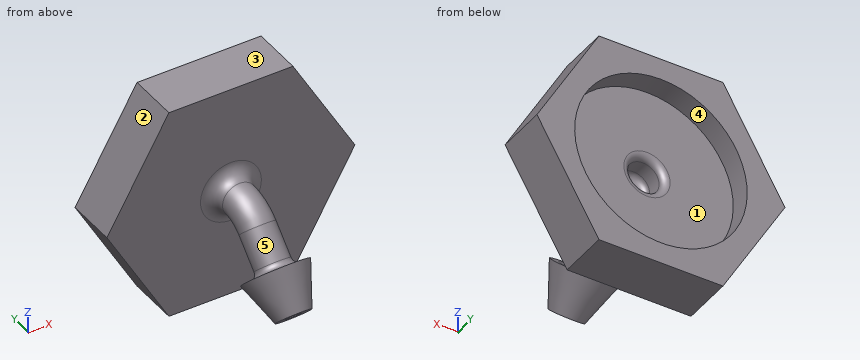
```python
from build123d import *

# Parameters (mm, degrees)
MAINHOLDER_DEPTH   = 7.5
SKETCH12_R         = 12.75
MAGNETCUTOUT_DEPTH = 3.28
MAGNETHOLE_REACH   = 26.614
SKETCH13_R         = 2.415
DRAINOPENING_R     = 2.5
DRAINOPENING_R_2   = 1.125
DRAINBASEFILLET_R  = 2
BARBBASEFILLET_R   = 1
DRAINOPENFILLET_R  = 1
MAGNETFILLET_R     = 1


with BuildPart() as part:
    # Sketch11 → MainHolder (new body)
    with BuildSketch(Plane(origin=(0, 0, 0), x_dir=(1, 0, 0), z_dir=(0, 1, 0))):
        Polygon((18.330871047, 0), (9.165435523, 15.875), (-9.165435523, 15.875), (-18.330871047, 0), (-9.165435523, -15.875), (9.165435523, -15.875), align=None)
    extrude(amount=MAINHOLDER_DEPTH)

    # Sketch12 → MagnetCutout (cut)
    with BuildSketch(Plane(origin=(0, 7.5, 0), x_dir=(1, 0, 0), z_dir=(0, 1, 0))):
        with Locations(Location((0, 0, 0), (0, 0, 270))):
            Circle(SKETCH12_R)
    extrude(amount=-MAGNETCUTOUT_DEPTH, mode=Mode.SUBTRACT)

    # Sketch13 → MagnetHole (cut, up to next)
    with BuildSketch(Plane(origin=(0, 4.22, 0), x_dir=(1, 0, 0), z_dir=(0, 1, 0)), mode=Mode.PRIVATE) as magnethole_sk1:
        with Locations(Location((0, 0, 0), (0, 0, 270))):
            Circle(SKETCH13_R)
    magnethole_tool1 = extrude(magnethole_sk1.sketch, amount=-MAGNETHOLE_REACH, mode=Mode.PRIVATE) & part.part
    add(magnethole_tool1.solids().sort_by_distance((0, 4.22, 0))[0], mode=Mode.SUBTRACT)

    # Drain: sweep along a path in DrainPath
    with BuildLine(Plane(origin=(0, 0, 0), x_dir=(0, 0, -1), z_dir=(1, 0, 0))) as drain_path:
        Line((0, 0), (0, -2))
        ThreePointArc((0, -2), (0.456722805, -4.296100594), (1.757359313, -6.242640687))
        Line((1.757359313, -6.242640687), (10.242640687, -14.727922061))
    # DrainOpening → Drain (sweep)
    with BuildSketch(Plane.XZ):
        Circle(DRAINOPENING_R)
        Circle(DRAINOPENING_R_2, mode=Mode.SUBTRACT)
    sweep(path=drain_path.line)

    # BarbOutline → Barb (revolve)
    with BuildSketch(Plane(origin=(0, 0, 0), x_dir=(0, -0.7071067811865461, -0.7071067811865489), z_dir=(-1, 0, 0)), mode=Mode.PRIVATE) as barb_sk:
        Polygon((17.656854249, 0.671572875), (11.656854249, 0.671572875), (11.656854249, -1.578427125), align=None)
    revolve(barb_sk.sketch.rotate(Axis((0, -5.447145558, -0.961864184), (0, -0.7071067811865461, -0.707106781186549)), 180), axis=Axis((0, -5.447145558, -0.961864184), (0, -0.7071067811865461, -0.707106781186549)))

    # DrainBaseFillet
    drainbasefillet_edges = [part.edges().sort_by_distance(p)[0] for p in [
        (-2.5, 0, 0),
    ]]
    fillet(drainbasefillet_edges, radius=DRAINBASEFILLET_R - 0.0001)  # a hair under: the kernel refuses the full size

    # BarbBaseFillet
    barbbasefillet_edges = [part.edges().sort_by_distance(p)[0] for p in [
        (-2.5, -10.485281374, -6),
    ]]
    fillet(barbbasefillet_edges, radius=BARBBASEFILLET_R)

    # DrainOpenFillet
    drainopenfillet_edges = [part.edges().sort_by_distance(p)[0] for p in [
        (0, 0, -2.415),
    ]]
    fillet(drainopenfillet_edges, radius=DRAINOPENFILLET_R)

    # MagnetFillet
    magnetfillet_edges = [part.edges().sort_by_distance(p)[0] for p in [
        (0, 4.22, -2.415),
    ]]
    fillet(magnetfillet_edges, radius=MAGNETFILLET_R)


solid = part.part
```
Design review of the part built by this model. Coordinates are the model's own, in mm. Face numbers are marked on the shaded views. A direction names the side the tool comes from. Give positions to 0.01 mm unless a question says otherwise; leave off trailing zeros. Order: outer loops, then holes, each group sorted by start corner. A loop starts at its lowest first (then second) coordinate and runs counter-clockwise, first axis right, second up. Notation, with made-up numbers: M 30.25,86.5 L 68.25,86.5 A32 ccw 68.25,122.5 Z; hole C 59,-36 d9. An arc over 180 degrees is marked long. One line per question, with ' | ' between items. Start each with the question number.
Q1. For pin 1 Ø4.5 at (x, z) = (0, 0) entering from -Y; pin 2 Ø2 at (x, z) = (0, 0) entering from -Y; pin 3 Ø2.5 at (x, z) = (-0.5, 0) entering from +Y, all flat-tipped, find the tip position at first contact; note any pin that passes through.
Q2. We need section D-D (y = -1). Write out the cut boundary in (x, z) (3 decimals).
Q3. We need section B-B (z = 6). Write out the cut boundary in (x, y).
Q4. We need section C-C (x = -8). Write out the cut boundary in (y, z) (3 decimals), plus the area to 3 significant figures.
Q5. The part is to be moulded in two halves that separate along X. For the marked faces 3, 4 and 5, say which applies: +X half, -X half, draft (parallel to the pull), parting line (faces both ways), or undercut.
Q6. We need section A-A (y = 2.75). Write out the cut boundary in (x, z) (3 decimals).
Q7. For L1, parallel to Y at x = -9, z = 2; L2, parallel to Y at x = 6, z = -12; L3, parallel to X at y = 6.2, z = 0, list the stretches that pass through material, from the lowest coordinate up. Write a range as [from, to].
Q8. Machinability: for the marked faces 1 and 2, which of the approach directions +Z, -Z, +X, -X, +Y, -Y give a long, thin tool a straight path to every point of the face, cutting with its end or side? Answer none if there is none.
Returned:
1) pin 1: y = -10.27 | pin 2: y = -9.02 | pin 3: y = 0.06
2) outline: C 0,0 d5.536; hole C 0,0 d2.25
3) outline: M -14.87,0 L 14.87,0 L 14.87,7.5 L 11.25,7.5 L 11.25,4.22 L -11.25,4.22 L -11.25,7.5 L -14.87,7.5 Z
4) outline: M 0,-15.875 L 7.5,-15.875 L 7.5,-9.928 L 4.22,-9.928 L 4.22,9.928 L 7.5,9.928 L 7.5,15.875 L 0,15.875 Z | area: 173 mm2
5) face 3: draft | face 4: undercut | face 5: parting line
6) outline: M -18.331,0 L -9.165,-15.875 L 9.165,-15.875 L 18.331,0 L 9.165,15.875 L -9.165,15.875 Z; hole C 0,0 d4.83
7) L1: [0, 4.22] | L2: [0, 7.5] | L3: [-18.33, -12.75], [12.75, 18.33]
8) face 1: +Y | face 2: +Z, -X, +Y, -Y
